Source: three-view drawing plus pictorial views. Frame: mm from the lowest corner of the part. Give positions to 0.01 mm unless a question says otherwise; leave off trailing zeros. Write each loop counter-clockwise with the first axis right and the second up, starting at its lowest first coordinate (ties: lowest second). Pieces come first, ordered by that corner, then holes. Notation, with made-up numbers: (-34.75, 67.25) -> (-27.75, 67.25) arc R20 ccw to (-27.75, 81.25) -> close; hole circle Ø9 at (62.25, 10.5). An arc over 180 degrees is marked (long way). Write item = value, one per line.
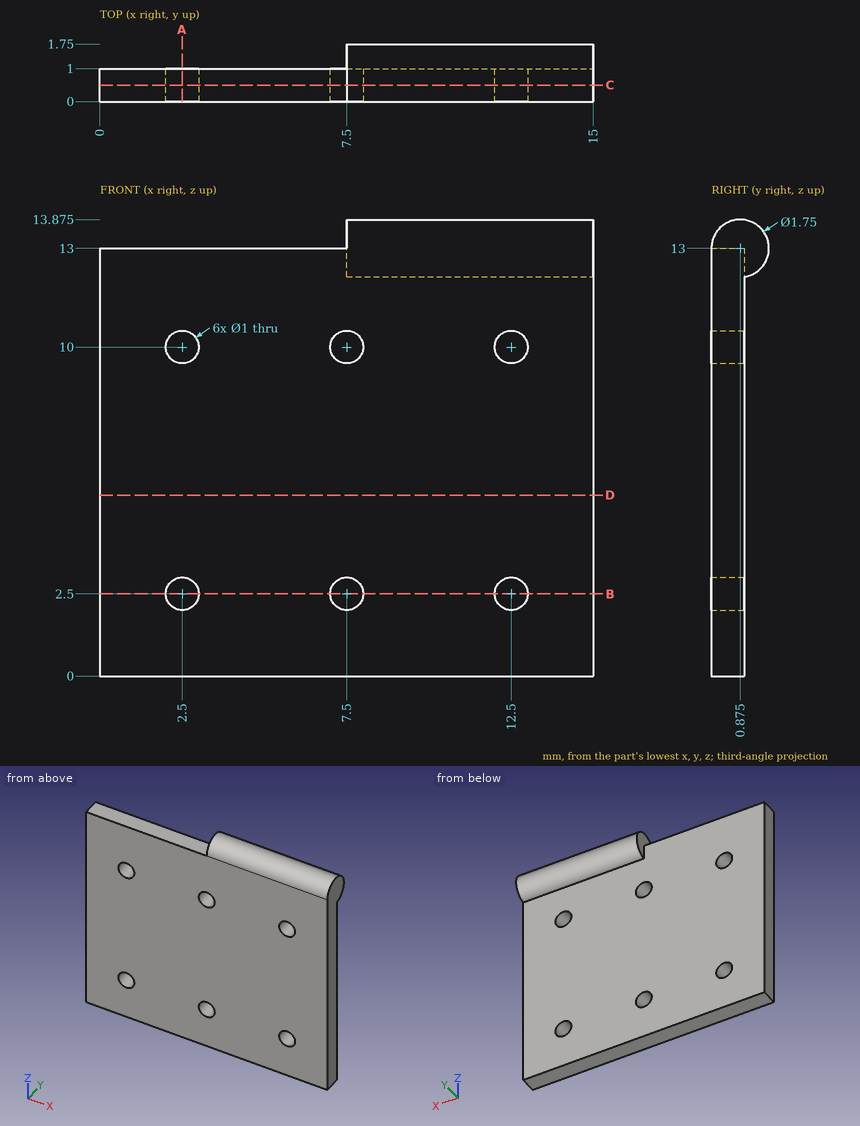
1) Cut plane A-A (x = 2.5). Return the cut outline in (y, z), then the cut area to 3 significant figures.
Computed:
outline = (0, 0) -> (1, 0) -> (1, 2) -> (0, 2) -> close; (0, 3) -> (1, 3) -> (1, 9.5) -> (0, 9.5) -> close; (0, 10.5) -> (1, 10.5) -> (1, 13) -> (0, 13) -> close
area = 11.0 mm²
2) Cut plane C-C (y = 0.5). Return the cut outline in (x, z).
Computed:
outline = (0, 0) -> (15, 0) -> (15, 13.79) -> (7.5, 13.79) -> (7.5, 13) -> (0, 13) -> close; hole circle Ø1 at (2.5, 2.5); hole circle Ø1 at (2.5, 10); hole circle Ø1 at (7.5, 2.5); hole circle Ø1 at (7.5, 10); hole circle Ø1 at (12.5, 2.5); hole circle Ø1 at (12.5, 10)
3) Cut plane B-B (z = 2.5). Return the cut outline in (x, y), then the cut area to 3 significant figures.
Computed:
outline = (0, 0) -> (2, 0) -> (2, 1) -> (0, 1) -> close; (3, 0) -> (7, 0) -> (7, 1) -> (3, 1) -> close; (8, 0) -> (12, 0) -> (12, 1) -> (8, 1) -> close; (13, 0) -> (15, 0) -> (15, 1) -> (13, 1) -> close
area = 12.0 mm²
4) Material intervals for L1, parallel to X at y = 0.4, z = 2.5; L2, parallel to Z at x = 2.5, y = 0.35; L3, parallel to Z at x = 12.5, y = 0.6, sorted ascending.
Computed:
L1 = 0 to 2, 3 to 7, 8 to 12, 13 to 15
L2 = 0 to 2, 3 to 9.5, 10.5 to 13
L3 = 0 to 2, 3 to 9.5, 10.5 to 13.83
5) Cut plane D-D (z = 5.5). Return the cut outline in (x, y).
Computed:
outline = (0, 0) -> (15, 0) -> (15, 1) -> (0, 1) -> close
